Source: CAD feature listing. Evaluate the final solid. Frame: model axes, mm. Face numbers are marked on the shaded views. A direction names the side the tool comes from. Give positions to 0.01 mm unless a question says otherwise; leave off trailing zeros. Write each loop counter-clockwise with the first axis right and the second up, starting at its lowest first coordinate (ties: lowest second). Pieces come first, ordered by that corner, then holes. Notation, with made-up numbers: M 72,-37 L 108,-37 A21 ccw 108,-1 Z; hole C -11,-19.75 d1. An arc over 180 degrees is marked long. Answer as a JSON object with one key per item and string values. Group by question number.
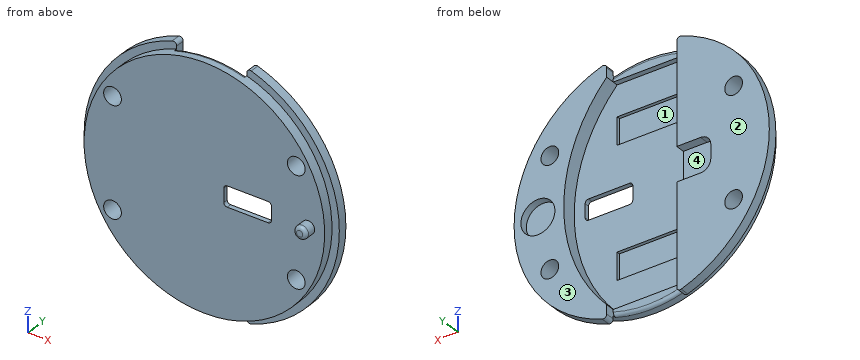
```python
from build123d import *

# Parameters (mm, degrees)
SKETCH1_R           = 35.35
SKETCH1_R_2         = 2.6
SKETCH1_W           = 14
SKETCH1_H           = 6
BOSS_EXTRUDE1_DEPTH = 1.4
FILLET1_R           = 1
SKETCH3_R           = 35.35
SKETCH3_R_2         = 2.6
BOSS_EXTRUDE3_DEPTH = 1.6
SKETCH4_R           = 2.6
BOSS_EXTRUDE4_DEPTH = 2.7
SKETCH5_R           = 5
CUT_EXTRUDE1_DEPTH  = 2.2
SKETCH7_W           = 20.6
SKETCH7_H           = 8
CUT_EXTRUDE3_DEPTH  = 1
SKETCH8_R           = 1.9
BOSS_EXTRUDE6_DEPTH = 3.5
FILLET2_R           = 1
FILLET3_R           = 3


with BuildPart() as part:
    # Sketch1 → Boss-Extrude1 (new body)
    with BuildSketch(Plane(origin=(0, 0, 0), x_dir=(1, 0, 0), z_dir=(0, 1, 0))):
        with Locations(Location((0, 0, 0), (0, 0, 270))):
            Circle(SKETCH1_R)
        with Locations(Location((27, 16, 0), (0, 0, 270))):
            Circle(SKETCH1_R_2, mode=Mode.SUBTRACT)
        with Locations(Location((-27, 16, 0), (0, 0, 270))):
            Circle(SKETCH1_R_2, mode=Mode.SUBTRACT)
        with Locations(Location((-27, -16, 0), (0, 0, 270))):
            Circle(SKETCH1_R_2, mode=Mode.SUBTRACT)
        with Locations(Location((27, -16, 0), (0, 0, 270))):
            Circle(SKETCH1_R_2, mode=Mode.SUBTRACT)
        with Locations((12.7, 0)):
            Rectangle(SKETCH1_W, SKETCH1_H, mode=Mode.SUBTRACT)
    extrude(amount=BOSS_EXTRUDE1_DEPTH)

    # Fillet1
    fillet1_edges = [part.edges().sort_by_distance(p)[0] for p in [
        (5.7, 0.7, -3),
        (5.7, 0.7, 3),
        (19.7, 0.7, 3),
        (19.7, 0.7, -3),
    ]]
    fillet(fillet1_edges, radius=FILLET1_R)

    # Sketch3 → Boss-Extrude3 (add)
    with BuildSketch(Plane(origin=(0, 1.4, 0), x_dir=(1, 0, 0), z_dir=(0, 1, 0))):
        with Locations(Location((0, 0, 0), (0, 0, 270))):
            Circle(SKETCH3_R)
        with Locations(Location((27, 16, 0), (0, 0, 270))):
            Circle(SKETCH3_R_2, mode=Mode.SUBTRACT)
        with Locations(Location((27, -16, 0), (0, 0, 270))):
            Circle(SKETCH3_R_2, mode=Mode.SUBTRACT)
        with Locations(Location((-27, -16, 0), (0, 0, 270))):
            Circle(SKETCH3_R_2, mode=Mode.SUBTRACT)
        with Locations(Location((-27, 16, 0), (0, 0, 270))):
            Circle(SKETCH3_R_2, mode=Mode.SUBTRACT)
        with BuildLine():
            Line((-10.3, 32.05), (10.3, 32.05))
            ThreePointArc((10.3, 32.05), (22.922718258, 0), (10.3, -32.05))
            Line((10.3, -32.05), (-10.3, -32.05))
            Line((-10.3, -32.05), (-10.3, 32.05))
        make_face(mode=Mode.SUBTRACT)
    extrude(amount=BOSS_EXTRUDE3_DEPTH)

    # Sketch4 → Boss-Extrude4 (add)
    # profile 1 of 2: a face of its own
    with BuildSketch(Plane(origin=(0, 3, 0), x_dir=(1, 0, 0), z_dir=(0, 1, 0))):
        with BuildLine():
            Line((-10.3, 36.057731487), (-10.3, 5))
            Line((-10.3, 5), (-20.3, 5))
            Line((-20.3, 5), (-20.3, -5))
            Line((-20.3, -5), (-10.3, -5))
            Line((-10.3, -5), (-10.3, -36.057731487))
            ThreePointArc((-10.3, -36.057731487), (-37.5, 0), (-10.3, 36.057731487))
        make_face()
        with Locations(Location((-27, 16, 0), (0, 0, 270))):
            Circle(SKETCH4_R, mode=Mode.SUBTRACT)
        with Locations(Location((-27, -16, 0), (0, 0, 270))):
            Circle(SKETCH4_R, mode=Mode.SUBTRACT)
    # profile 2 of 2: a face of its own
    with BuildSketch(Plane(origin=(0, 3, 0), x_dir=(1, 0, 0), z_dir=(0, 1, 0))):
        with BuildLine():
            Line((10.3, 32.05), (10.3, 36.057731487))
            ThreePointArc((10.3, 36.057731487), (37.5, 0), (10.3, -36.057731487))
            Line((10.3, -36.057731487), (10.3, -32.05))
            ThreePointArc((10.3, -32.05), (22.922718258, 0), (10.3, 32.05))
        make_face()
        with Locations(Location((27, -16, 0), (0, 0, 270))):
            Circle(SKETCH4_R, mode=Mode.SUBTRACT)
        with Locations(Location((27, 16, 0), (0, 0, 270))):
            Circle(SKETCH4_R, mode=Mode.SUBTRACT)
    extrude(amount=BOSS_EXTRUDE4_DEPTH)

    # Sketch5 → Cut-Extrude1 (cut)
    with BuildSketch(Plane(origin=(0, 5.7, 0), x_dir=(1, 0, 0), z_dir=(0, 1, 0))):
        with Locations(Location((30.5, 0, 0), (0, 0, 270))):
            Circle(SKETCH5_R)
    extrude(amount=-CUT_EXTRUDE1_DEPTH, mode=Mode.SUBTRACT)

    # Sketch7 → Cut-Extrude3 (cut)
    with BuildSketch(Plane(origin=(0, 1.4, 0), x_dir=(1, 0, 0), z_dir=(0, 1, 0))):
        with Locations((0, -19.05)):
            Rectangle(SKETCH7_W, SKETCH7_H)
        with Locations((0, 19.05)):
            Rectangle(SKETCH7_W, SKETCH7_H)
    extrude(amount=-CUT_EXTRUDE3_DEPTH, mode=Mode.SUBTRACT)

    # Sketch8 → Boss-Extrude6 (add)
    with BuildSketch(Plane.XZ):
        with Locations(Location((30.5, 0, 0), (0, 0, 90))):
            Circle(SKETCH8_R)
    extrude(amount=BOSS_EXTRUDE6_DEPTH)

    # Fillet2
    # the kernel refuses this fillet: 1 mm, written as the material it takes off along each edge
    with BuildSketch(Plane(origin=(0, 3, 0), x_dir=(0, 0, 1), z_dir=(-1, 0, 0))) as fillet2_piece_1_section:
        with BuildLine():
            CenterArc((35.35 - FILLET2_R, -FILLET2_R), FILLET2_R, 0, 90)
            Line((35.35 - FILLET2_R, 0), (35.35, 0))
            Line((35.35, 0), (35.35, -FILLET2_R))
        make_face()
    fillet2_piece_1 = revolve(axis=Axis((0, 3, 0), (0, 1, 0)), revolution_arc=20.992206164, mode=Mode.PRIVATE)
    fillet2_piece_1 = split(fillet2_piece_1, bisect_by=Plane(origin=(10.3, 2.776649723, 34.610378642), z_dir=(-1, 0, 0)), keep=Keep.TOP, mode=Mode.PRIVATE)
    add(fillet2_piece_1, mode=Mode.SUBTRACT)
    with BuildSketch(Plane(origin=(-10.3, -0.42335266, -36.057731487), x_dir=(0, 0, 1), z_dir=(0, 1, 0)), Plane(origin=(10.3, -0.42335266, 36.057731487), x_dir=(0, 0, -1), z_dir=(0, 1, 0))) as fillet2_piece_2:
        with BuildLine():
            CenterArc((1.350959814, -1), FILLET2_R, 90, 108.034465952)
            ThreePointArc((0.400089357, -1.309589041), (0.1940666, -0.656620869), (0, 0))
            Line((0, 0), (1.350959814, 0))
        make_face()
    extrude(amount=9.546705321, mode=Mode.SUBTRACT)
    with BuildSketch(Plane(origin=(-10.3, -0.42335266, 36.057731487), x_dir=(0, 0, -1), z_dir=(0, 1, 0)), Plane(origin=(10.3, -0.42335266, -36.057731487), x_dir=(0, 0, 1), z_dir=(0, 1, 0))) as fillet2_piece_3:
        with BuildLine():
            CenterArc((1.350959814, 1), FILLET2_R, 161.965534048, 108.034465952)
            ThreePointArc((0.400089357, 1.309589041), (0.1940666, 0.656620869), (0, 0))
            Line((0, 0), (1.350959814, 0))
        make_face()
    extrude(amount=9.546705321, mode=Mode.SUBTRACT)
    with BuildSketch(Plane(origin=(30.5, -3.5, 0), x_dir=(0, 0, 1), z_dir=(1, 0, 0))) as fillet2_piece_4:
        with BuildLine():
            CenterArc((1.9 - FILLET2_R, -FILLET2_R), FILLET2_R, 0, 90)
            Line((1.9 - FILLET2_R, 0), (1.9, 0))
            Line((1.9, 0), (1.9, -FILLET2_R))
        make_face()
    revolve(axis=Axis((30.5, -3.5, 0), (0, -1, 0)), mode=Mode.SUBTRACT)
    with BuildSketch(Plane(origin=(0, 3, 0), x_dir=(0.3582437714618883, 0, -0.9336280845222912), z_dir=(0.9336280845222912, 0, 0.3582437714618883))) as fillet2_piece_5_section:
        with BuildLine():
            CenterArc((35.35 - FILLET2_R, -FILLET2_R), FILLET2_R, 0, 90)
            Line((35.35 - FILLET2_R, 0), (35.35, 0))
            Line((35.35, 0), (35.35, -FILLET2_R))
        make_face()
    fillet2_piece_5 = revolve(axis=Axis((0, 3, 0), (0, 1, 0)), revolution_arc=41.984758253, mode=Mode.PRIVATE)
    fillet2_piece_5 = split(fillet2_piece_5, bisect_by=Plane(origin=(-10.3, 2.718769388, -35.068769388), z_dir=(1, 0, 0)), keep=Keep.TOP, mode=Mode.PRIVATE)
    fillet2_piece_5 = split(fillet2_piece_5, bisect_by=Plane(origin=(10.3, 2.718769388, -35.068769388), z_dir=(-1, 0, 0)), keep=Keep.TOP, mode=Mode.PRIVATE)
    add(fillet2_piece_5, mode=Mode.SUBTRACT)
    with BuildSketch(Plane(origin=(0, 3, 0), x_dir=(-0.35824095305440445, 0, 0.9336291659725889), z_dir=(-0.9336291659725889, 0, -0.35824095305440445))) as fillet2_piece_6_section:
        with BuildLine():
            CenterArc((35.35 - FILLET2_R, -FILLET2_R), FILLET2_R, 0, 90)
            Line((35.35 - FILLET2_R, 0), (35.35, 0))
            Line((35.35, 0), (35.35, -FILLET2_R))
        make_face()
    fillet2_piece_6 = revolve(axis=Axis((0, 3, 0), (0, 1, 0)), revolution_arc=20.992206164, mode=Mode.PRIVATE)
    fillet2_piece_6 = split(fillet2_piece_6, bisect_by=Plane(origin=(-10.3, 2.776650175, 34.610378573), z_dir=(1, 0, 0)), keep=Keep.TOP, mode=Mode.PRIVATE)
    add(fillet2_piece_6, mode=Mode.SUBTRACT)

    # Fillet3
    fillet3_edges = [part.edges().sort_by_distance(p)[0] for p in [
        (-20.3, 4.35, 5),
        (-20.3, 4.35, -5),
    ]]
    fillet(fillet3_edges, radius=FILLET3_R)


solid = part.part
```
(1) Section A-A, the plane x = 15.5. Return loops of the section in (y, z), plus the area to 3 significant figures.
(2) Ray query, L1, parallel to X at y = 3.8, z = -16; L2, parallel to X at y = 2.45, z = 16; L3, parallel to Z at x = -28.5, y = 4.25. Return the intervals inside material, ascending. Write a range as [from, to].
(3) Access query for the marked faces 3 and 4. Directions: +Z, -Z, +X, -X, +Y, -Y. A direction counts if a zero-diameter tool reaches every point of the face in a straight line with its end or side. Return the directions, or none.
(4) Section B-B, the plane z = -16. Return loops of the section in (x, y), plus the area to 3 significant figures.
(5) Pull-direction query (Z, two-part tool) for the marked faces 1 and 2; classes: pulls with the +Z half, pulls with the -Z half, needs draft (parallel to the pull), parting line crosses it, or undercut.
(6) Contact query for flat-ended pins moving along their axis: pin 1 Ø10 at (x, z) = (19.5, 0) entering from +Y; pin 2 Ø3 at (x, y) = (15.5, 1) entering from -Z; pin 3 Ø8 at (x, z) = (-20, -23.5) entering from -Y; pin 4 Ø8 at (x, z) = (-15.5, -0.5) entering from +Y. Output: stop coordinate, or through.
(7) Section C-C, the plane x = -27. Return loops of the section in (y, z).
(8) Section D-D, the plane z = -26. Return loops of the section in (x, y).
Reported:
{
 "1": {"outline": "M 0,-31.77 L 3,-31.77 L 3,-34.15 L 5.7,-34.15 L 5.7,-25.35 L 1.4,-25.35 L 1.4,-3 L 0,-3 Z; M 0,3 L 1.4,3 L 1.4,25.35 L 5.7,25.35 L 5.7,34.15 L 3,34.15 L 3,31.77 L 0,31.77 Z", "area": "149 mm2"},
 "2": {"L1": "x = [-33.92, -29.6], [-24.4, -10.3], [20.12, 24.4], [29.6, 33.92]", "L2": "x = [-31.52, -29.6], [-24.4, -10.3], [20.12, 24.4], [29.6, 31.52]", "L3": "z = [-24.37, -18.12], [-13.88, 13.88], [18.12, 24.37]"},
 "3": {"face 3": "+Z, -Z, +X, -X, +Y", "face 4": "+Y"},
 "4": {"outline": "M -33.92,3 L -31.52,3 L -31.52,0 L -29.6,0 L -29.6,5.7 L -33.92,5.7 Z; M -24.4,0 L 24.4,0 L 24.4,5.7 L 20.12,5.7 L 20.12,1.4 L 10.3,1.4 L 10.3,0.4 L -10.3,0.4 L -10.3,5.7 L -24.4,5.7 Z; M 29.6,0 L 31.52,0 L 31.52,3 L 33.92,3 L 33.92,5.7 L 29.6,5.7 Z", "area": "162 mm2"},
 "5": {"face 1": "undercut", "face 2": "needs draft"},
 "6": {"pin 1": "stops at y = 5.7", "pin 2": "stops at z = -32.46", "pin 3": "stops at y = 0", "pin 4": "stops at y = 3"},
 "7": {"outline": "M 0,-22.82 L 3,-22.82 L 3,-26.02 L 5.7,-26.02 L 5.7,-18.6 L 0,-18.6 Z; M 0,-13.4 L 5.7,-13.4 L 5.7,13.4 L 0,13.4 Z; M 0,18.6 L 5.7,18.6 L 5.7,26.02 L 3,26.02 L 3,22.82 L 0,22.82 Z"},
 "8": {"outline": "M -27.02,3 L -23.95,3 L -23.95,0 L 23.95,0 L 23.95,3 L 27.02,3 L 27.02,5.7 L 15.08,5.7 L 15.08,1.4 L -10.3,1.4 L -10.3,5.7 L -27.02,5.7 Z"}
}
